Check sheet for the modelled part. Datum: model origin and axes. Units: mm. A direction names the side the tool comes from. Coordinates: 2 decimals unless noted, no trailing zeros. Order: outer loops, then holes, each group sorted by start corner. A loop starts at its lowest first (then second) coordinate and runs counter-clockwise, first axis right, second up.
Autodesk Inventor part; units mm, degrees
ref_plane "YZ Plane" through (0, 0, 0) normal (1, 0, 0) x (0, 1, 0)
ref_plane "XZ Plane" through (0, 0, 0) normal (0, 1, 0) x (-1, 0, 0)
ref_plane "XY Plane" through (0, 0, 0) normal (0, 0, 1) x (1, 0, 0)
sketch "Szkic1" plane through (0, 0, 0) normal (0, 1, 0) x (-1, 0, 0)
  line L0 (21, 21) -> (-21, 21)
  line L1 (-21, 21) -> (-21, -21)
  line L2 (-21, -21) -> (21, -21)
  line L3 (21, -21) -> (21, 21)
  line L4 (21, 21) -> (-21, -21)
  line L5 (21, -21) -> (-21, 21)
  point P0 (0, 0)
  point P1 (0, 0)
  dimension "d0" = 42
  dimension "d1" = 42
extrude "Wyciągnięcie proste1" add sketch "Szkic1" along normal blind 40
sketch "Szkic2" plane through (0, 40, 0) normal (0, 1, 0) x (1, 0, 0)
  circle A0 centre (0, 0) radius 2.5
  dimension "d4" = 5
extrude "Wyciągnięcie proste2" add sketch "Szkic2" along normal blind 24
properties part number "Stepper_model"
(1) Thickness scan on probe 1 along Y at (x, z) = (1, -17). Record the ranges inside material, lowest first.
Filled in:
probe 1: y = 0 to 40
(2) Cross-section at A-A (z = 0). Enter the section's corners in (x, y).
Filled in:
outline: (-21, 0) - (21, 0) - (21, 40) - (2.5, 40) - (2.5, 64) - (-2.5, 64) - (-2.5, 40) - (-21, 40) - close
(3) Cross-section at D-D (z = -5.5). Enter the section's corners in (x, y).
Filled in:
outline: (-21, 0) - (21, 0) - (21, 40) - (-21, 40) - close
(4) Go/stop test with flat-tipped pins: P1, Ø1, axis at x = -9.5, z = 1, coming from the +Y side; P2, Ø12.5, axis at x = -3.5, z = -2, coming from the +Y side. Record where each tip stops, or that it passes through.
Filled in:
P1: stops at y = 40
P2: stops at y = 64
(5) Cross-section at B-B (x = 0). Enter the section's corners in (y, z), and give its area (3 significant figures).
Filled in:
outline: (0, -21) - (40, -21) - (40, -2.5) - (64, -2.5) - (64, 2.5) - (40, 2.5) - (40, 21) - (0, 21) - close
area: 1,800 mm2
(6) Cross-section at C-C (x = 5). Enter the section's corners in (y, z), and give its area (3 significant figures).
Filled in:
outline: (0, -21) - (40, -21) - (40, 21) - (0, 21) - close
area: 1,680 mm2
(7) Tool access check on faces 1 (the cylindrical face through (-0.54, 51.83, -2.44)), 2 (the flat face through (-21, 20, 0)). Record the directions out of +Z, -Z, +X, -X, +Y, -Y that give a thin tool (end or side, any length) a straight path to the whole face; none if there is none.
Filled in:
face 1: +Y
face 2: +Z, -Z, -X, +Y, -Y
